```python
from build123d import *

# Parameters (mm, degrees)
F1_DEPTH = 25
F2_R     = 12.5
F3_DEPTH = 2
F4_R     = 3.5
F5_DEPTH = 6
F6_SIZE  = 5
F8_DEPTH = 15


with BuildPart() as f1:
    # F0 (on Top) → F1 (new body)
    with BuildSketch(Plane.XY):
        with BuildLine():
            Line((17.320508, 30), (-17.320508, 30))
            ThreePointArc((-17.320508, 30), (-34.641016, 20), (-34.641016, 0))
            Line((-34.641016, 0), (-17.320508, -30))
            ThreePointArc((-17.320508, -30), (0, -40), (17.320508, -30))
            Line((17.320508, -30), (34.641016, 0))
            ThreePointArc((34.641016, 0), (34.641016, 20), (17.320508, 30))
        make_face()
    extrude(amount=F1_DEPTH)

    # F2 (on face) → F3 (cut)
    with BuildSketch(Plane.XY.offset(25)):
        with Locations((-17.320508, 10)):
            Circle(F2_R)
        with Locations((0, -20)):
            Circle(F2_R)
        with Locations((17.320508, 10)):
            Circle(F2_R)
    extrude(amount=-F3_DEPTH, mode=Mode.SUBTRACT)

    # F4 (on face) → F5 (cut)
    with BuildSketch(Plane.XY.offset(23)):
        with Locations((-17.320508, 10)):
            Circle(F4_R)
        with Locations((0, -20)):
            Circle(F4_R)
        with Locations((17.320508, 10)):
            Circle(F4_R)
    extrude(amount=-F5_DEPTH, mode=Mode.SUBTRACT)

    # F6
    f6_edges = [f1.edges().sort_by_distance(p)[0] for p in [
        (25.980762, -15, 25),
    ]]
    chamfer(f6_edges, length=F6_SIZE)

    # F7 (on face) → F8 (cut)
    with BuildSketch(Plane(origin=(0, 0, 0), x_dir=(1, 0, 0), z_dir=(0, 0, -1))):
        with BuildLine():
            ThreePointArc((12.990381, 27.5), (0, 35), (-12.990381, 27.5))
            Line((-12.990381, 27.5), (-30.310889, -2.5))
            ThreePointArc((-30.310889, -2.5), (-30.310889, -17.5), (-17.320508, -25))
            Line((-17.320508, -25), (17.320508, -25))
            ThreePointArc((17.320508, -25), (30.310889, -17.5), (30.310889, -2.5))
            Line((30.310889, -2.5), (12.990381, 27.5))
        make_face()
    extrude(amount=-F8_DEPTH, mode=Mode.SUBTRACT)


solid = f1.part
```
Source: CAD feature listing. Evaluate the final solid. Frame: model axes, mm. A direction names the side the tool comes from. Coordinates: 2 decimals unless noted, no trailing zeros. Write each loop counter-clockwise with the first axis right and the second up, starting at its lowest first coordinate (ties: lowest second). Pieces come first, ordered by that corner, then holes. Notation, with made-up numbers: M 22.25,-22.75 L 34.25,-22.75 A17 ccw 34.25,4.25 Z; hole C 82.5,43.5 d10. An arc over 180 degrees is marked long. Answer as a JSON object with one key per item and string values.
1. Ray query, L1, parallel to Z at x = 7.5, y = 4.5; L2, parallel to Z at x = 1, y = 14; L3, parallel to X at y = 12, z = 7.5. Return the intervals inside material, ascending.
Evaluation:
{"L1": "15 to 23", "L2": "15 to 25", "L3": "-37.22 to -32.19, 32.19 to 37.22"}
2. Cut plane B-B on y = 10. Output: boundary loops of the cut face in (x, z).
Evaluation:
{"outline": "M -37.32,0 L -32.32,0 L -32.32,15 L 32.32,15 L 32.32,0 L 37.32,0 L 37.32,20 L 32.32,25 L 29.82,25 L 29.82,23 L 20.82,23 L 20.82,17 L 13.82,17 L 13.82,23 L 4.82,23 L 4.82,25 L -4.82,25 L -4.82,23 L -13.82,23 L -13.82,17 L -20.82,17 L -20.82,23 L -29.82,23 L -29.82,25 L -32.32,25 L -37.32,20 Z"}
3. Access query for faces 1 (the flat face through (-21.53, -12.71, 7.4)), 2 (the flat face through (3, -23, 23)), 3 (the flat face through (25.86, -15.21, 9.86)). Directions: +Z, -Z, +X, -X, +Y, -Y. A direction counts if a zero-diameter tool reaches every point of the face in a straight line with its end or side. Return the directions, or none.
Evaluation:
{"face 1": "-Z", "face 2": "+Z", "face 3": "+Z, -Z, +X, -Y"}
4. Cut plane D-D on z = 21. Output: boundary loops of the cut face in (x, y) (1 decimal).
Evaluation:
{"outline": "M -33.8,0.5 L -16.5,-29.5 A19 ccw 16.5,-29.5 L 33.8,0.5 A19 ccw 17.3,29 L -17.3,29 A19 ccw Z; hole C -17.3,10 d7; hole C 0,-20 d7; hole C 17.3,10 d7"}
5. Draft query along X for faces 4 (the cylindrical face through (0, -40, 10)), 5 (the flat face through (0, 28, 22)), 6 (the cylindrical face through (34.786, 19.745, 9.86)), 7 (the flat face through (-17, 10, 17)). Return one class per face: released by +X, released by -X, zero draft, split by the parting line, or undercut.
Evaluation:
{"face 4": "split by the parting line", "face 5": "zero draft", "face 6": "released by +X", "face 7": "undercut"}
6. Cut plane C-C on x = 0. Output: boundary loops of the cut face in (y, z).
Evaluation:
{"outline": "M -40,0 L -35,0 L -35,15 L 25,15 L 25,0 L 30,0 L 30,20 L 25,25 L -7.5,25 L -7.5,23 L -16.5,23 L -16.5,17 L -23.5,17 L -23.5,23 L -32.5,23 L -32.5,25 L -35,25 L -40,20 Z"}
7. Contact query for flat-ended pins moving along their axis: P1, Ø4, axis at x = -17.32, y = 10, coming from the -Z side; P2, Ø8, axis at y = -10, z = 18.5, coming from the +X side; P3, Ø7.5, axis at x = 17, y = 9.5, coming from the +Z side. Output: stop coordinate, or through.
Evaluation:
{"P1": "z = 15", "P2": "x = 31.18", "P3": "z = 23"}
8. Cut plane A-A on z = 12. Output: boundary loops of the cut face in (x, y), plus the area to 3 significant figures.
Evaluation:
{"outline": "M -34.64,0 L -17.32,-30 A20 ccw 17.32,-30 L 34.64,0 A20 ccw 17.32,30 L -17.32,30 A20 ccw Z; hole M -30.31,2.5 L -12.99,-27.5 A15 ccw 12.99,-27.5 L 30.31,2.5 A15 ccw 17.32,25 L -17.32,25 A15 ccw Z", "area": "1,070 mm^2"}
